The listing builds one solid part. Answer for the finished solid, in the listing's coordinates (mm). A direction names the side the tool comes from. Round coordinates to 2 decimals unless told otherwise and drop trailing zeros. Loops run counter-clockwise (first coordinate to the right, second up) from the corner with the lowest first, then second, coordinate; pieces in that order, holes last. Notation, with made-up numbers: M 70.5,83.25 L 85.5,83.25 A10 ccw 85.5,99.25 Z; hole C 68,60 d8. An arc over 180 degrees is marked long. Put each result on its own line as item: value. Start each with the question number.
(1) Section D-D, the plane y = 19 is taken. Determine the outline of the cut face in (x, z).
(2) Flat-ended cylindrical pins translate along their axes: P1, Ø2, axis at x = 7.5, z = 2, coming from the -Y side; P2, Ø2, axis at x = -31, z = 1, coming from the +Y side; P3, Ø1.9, axis at y = 19, z = 3, coming from the -X side. Find the tip coordinate at first contact, or state that the pin passes through.
(3) Section B-B, the plane x = 2 is taken. Determine the outline of the cut face in (y, z).
(4) Which of the six approach directions +Z, -Z, +X, -X, +Y, -Y give full straight-line access (tool end or side, diameter ignored) to faces 1 (the face through (30.439, 18, 3)), 2 (the face through (-26.176, 20, 3)), 3 (the face through (2, 20.309, 3)), 4 (the face through (6.58, -2.45, 3.13)), 5 (the face through (-7, -3, 6.35))?
(5) Section A-A, the plane y = -3 is taken. Determine the outline of the cut face in (x, z).
(6) Determine the mould class of faces 6 (the face through (-16.783, -11.409, 3.131)), 7 (the face through (-32.4, -44.4, 3.1)), 8 (the face through (-7, -3, 0)) for opening direction Y: released by +Y, released by -Y, zero draft, split by the parting line, or undercut.
(7) Straight lines are drawn through the part: line 1 (X direction, y = 15.5, z = 6); line 2 (X direction, y = 23.5, z = 4.75); line 3 (Y direction, x = -3, z = 1). For each, find the intervals that lie inside material, in ascending order.
```python
from build123d import *

# Parameters (mm, degrees)
F1_DEPTH = 6.35


with BuildPart() as f1:
    # F0 (on Top) → F1 (new body)
    with BuildSketch(Plane.XY):
        with BuildLine():
            Line((-13.475527, 26.65859), (-26.175527, 26.65859))
            Line((-26.175527, 26.65859), (-26.175527, 13.95859))
            ThreePointArc((-26.175527, 13.95859), (-16.870071, -11.805035), (-36.482046, -30.929006))
            ThreePointArc((-36.482046, -30.929006), (-38.308198, -32.031301), (-39.024714, -34.040402))
            Line((-39.024714, -34.040402), (-39.024714, -44.193178))
            Line((-39.024714, -44.193178), (-39.024714, -56.90741))
            Line((-39.024714, -56.90741), (-32.674714, -56.90741))
            Line((-32.674714, -56.90741), (-32.674714, -45.69473))
            ThreePointArc((-32.674714, -45.69473), (-32.369919, -44.337325), (-31.514054, -43.240538))
            Line((-31.514054, -43.240538), (29.277846, 6.655949))
            ThreePointArc((29.277846, 6.655949), (30.133711, 7.752736), (30.438506, 9.110141))
            Line((30.438506, 9.110141), (30.438506, 26.65859))
            Line((30.438506, 26.65859), (17.738506, 26.65859))
            Line((17.738506, 26.65859), (17.738506, 23.48359))
            ThreePointArc((17.738506, 23.48359), (16.80857, 21.238526), (14.563506, 20.30859))
            Line((14.563506, 20.30859), (-10.300527, 20.30859))
            ThreePointArc((-10.300527, 20.30859), (-12.545591, 21.238526), (-13.475527, 23.48359))
            Line((-13.475527, 23.48359), (-13.475527, 26.65859))
        make_face()
        with BuildLine():
            ThreePointArc((-1.531554, -9.106644), (-4.993641, -9.478165), (-6.714508, -6.451172))
            ThreePointArc((-6.714508, -6.451172), (-7.107301, -0.531525), (-9.005287, 5.089344))
            ThreePointArc((-9.005287, 5.089344), (-8.847646, 8.166009), (-6.153785, 9.66061))
            Line((-6.153785, 9.66061), (12.460999, 9.66061))
            ThreePointArc((12.460999, 9.66061), (15.450371, 7.555321), (14.475339, 4.031418))
            Line((14.475339, 4.031418), (-1.531554, -9.106644))
        make_face(mode=Mode.SUBTRACT)
    extrude(amount=F1_DEPTH)


solid = f1.part
```
Recorded:
1. outline: M -26.18,0 L 30.44,0 L 30.44,6.35 L -26.18,6.35 Z
2. P1: stops at y = -12.04
2. P2: stops at y = -28.66
2. P3: stops at x = -26.18
3. outline: M -15.73,0 L -6.21,0 L -6.21,6.35 L -15.73,6.35 Z; M 9.66,0 L 20.31,0 L 20.31,6.35 L 9.66,6.35 Z
4. face 1: +Z, -Z, +X, +Y, -Y
4. face 2: +Z, -Z, -X, +Y
4. face 3: +Z, -Z, +Y
4. face 4: +Z, -Z
4. face 5: +Z, +X, -X, +Y, -Y
5. outline: M -16.43,0 L -6.76,0 L -6.76,6.35 L -16.43,6.35 Z; M 5.91,0 L 17.51,0 L 17.51,6.35 L 5.91,6.35 Z
6. face 6: undercut
6. face 7: released by -Y
6. face 8: zero draft
7. line 1: x = -26.18 to 30.44
7. line 2: x = -26.18 to -13.48, 17.74 to 30.44
7. line 3: y = -19.84 to -9.78, 9.66 to 20.31
